The drawing under review shows one solid part. Ordinate dimensions are in mm from its lowest x, y, z. A direction names the side the tool comes from. Coordinates: 2 decimals unless noted, no trailing zeros. Order: outer loops, then holes, each group sorted by start corner. A loop starts at its lowest first (then second) coordinate and runs counter-clockwise, first axis right, second up.
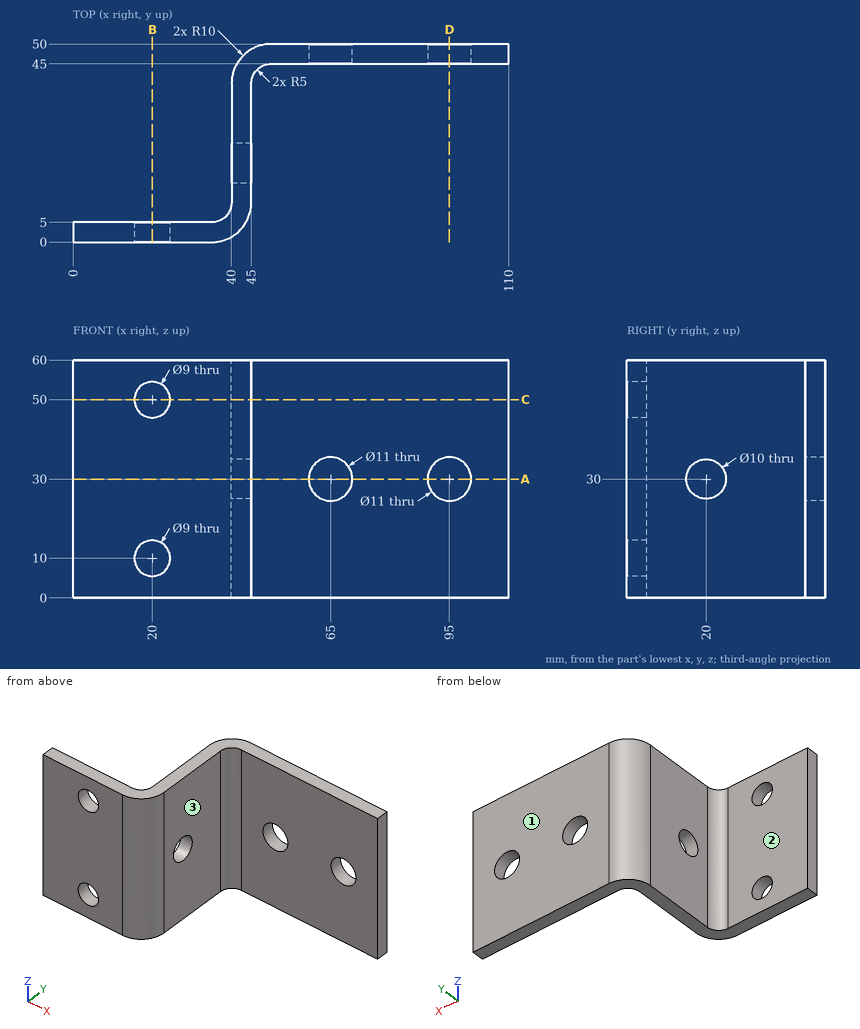
(1) We need section D-D, the plane x = 95. Write out the cut boundary in (y, z).
A:
outline: (45, 0) - (50, 0) - (50, 24.5) - (45, 24.5) - close; (45, 35.5) - (50, 35.5) - (50, 60) - (45, 60) - close
(2) We need section A-A, the plane z = 30. Write out the cut boundary in (x, y), and give its area (3 significant figures).
A:
outline: (0, 0) - (35, 0) arc R10 ccw to (45, 10) - (45, 15) - (40, 15) - (40, 10) arc R5 cw to (35, 5) - (0, 5) - close; (40, 25) - (45, 25) - (45, 40) arc R5 cw to (50, 45) - (59.5, 45) - (59.5, 50) - (50, 50) arc R10 ccw to (40, 40) - close; (70.5, 45) - (89.5, 45) - (89.5, 50) - (70.5, 50) - close; (100.5, 45) - (110, 45) - (110, 50) - (100.5, 50) - close
area: 583 mm2
(3) We need section B-B, the plane x = 20. Write out the cut boundary in (y, z), and give its area (3 significant figures).
A:
outline: (0, 0) - (5, 0) - (5, 5.5) - (0, 5.5) - close; (0, 14.5) - (5, 14.5) - (5, 45.5) - (0, 45.5) - close; (0, 54.5) - (5, 54.5) - (5, 60) - (0, 60) - close
area: 210 mm2
(4) Wall thickness on probe 1 along Z at (x, y) = (20, 2); probe 2 along Z at (x, y) = (65, 48.7); probe 3 along Y at (x, z) = (84, 52): over which ranges is each line inside the solid? List them lowest first.
A:
probe 1: z = 0 to 5.5, 14.5 to 45.5, 54.5 to 60
probe 2: z = 0 to 24.5, 35.5 to 60
probe 3: y = 45 to 50
(5) For pin 1 Ø1 at (y, z) = (20.5, 42.5) entering from -X; pin 2 Ø10.5 at (x, z) = (10.5, 39.5) entering from +Y; pin 3 Ø5.5 at (x, z) = (20, 10) entering from +Y; pin 4 Ø12 at (x, z) = (52.5, 46) entering from -Y, all flat-tipped, find the tip position at first contact; note any pin that passes through.
A:
pin 1: stops at x = 40
pin 2: stops at y = 5
pin 3: passes through
pin 4: stops at y = 43.57
(6) We need section C-C, the plane z = 50. Write out the cut boundary in (x, y), and give its area (3 significant figures).
A:
outline: (0, 0) - (15.5, 0) - (15.5, 5) - (0, 5) - close; (24.5, 0) - (35, 0) arc R10 ccw to (45, 10) - (45, 40) arc R5 cw to (50, 45) - (110, 45) - (110, 50) - (50, 50) arc R10 ccw to (40, 40) - (40, 10) arc R5 cw to (35, 5) - (24.5, 5) - close
area: 698 mm2
(7) Machinability: for the marked faces 1, 2 and 3, which of the approach directions +Z, -Z, +X, -X, +Y, -Y give a long, thin tool a straight path to every point of the face, cutting with its end or side? Answer none if there is none.
A:
face 1: +Z, -Z, +X, -X, +Y
face 2: +Z, -Z, -X, +Y
face 3: +Z, -Z, +X, -Y
